Design review of the part shown in the three views and the two pictorial views. Dimensions are in mm from the part's minimum x, y and z. A direction names the side the tool comes from. Round coordinates to 2 decimals unless told otherwise and drop trailing zeros. Loops run counter-clockwise (first coordinate to the right, second up) from the corner with the lowest first, then second, coordinate; pieces in that order, holes last.
1. Consider section A-A on y = 40.85. State the section outline as (x, z) points (3 decimals), then the cut area to 3 significant figures.
2. Consider section D-D on y = 24. State the section outline as (x, z) points, then the cut area to 3 significant figures.
3. Consider section C-C on z = 14.25. State the section outline as (x, y) points.
4. To check wall thickness, follow line 1 along Z through (x, y) = (1.85, 40.85) (3 decimals); line 2 along Z through (x, y) = (109, 2.5); line 3 along Y through (x, z) = (45, 3). State the ranges of each line that lie inside material, in increasing order.
5. Consider section B-B on x = 124. State the section outline as (y, z) points, then the cut area to 3 significant figures.
6. Clearance check with flat-ended pins moving along their axes: pin 1 Ø5 at (y, z) = (12.5, 17) entering from +X; pin 2 Ø4 at (x, y) = (152.5, 8) entering from +Z; pin 3 Ø3 at (x, z) = (37.5, 20.5) entering from +Y. State where each tip first meets the part, or that it passes through.
7. Tool access review of the marked faces 1 and 2: name each direction out of +Z, -Z, +X, -X, +Y, -Y from which nothing blocks a thin tool from reaching the whole face with its end or side.
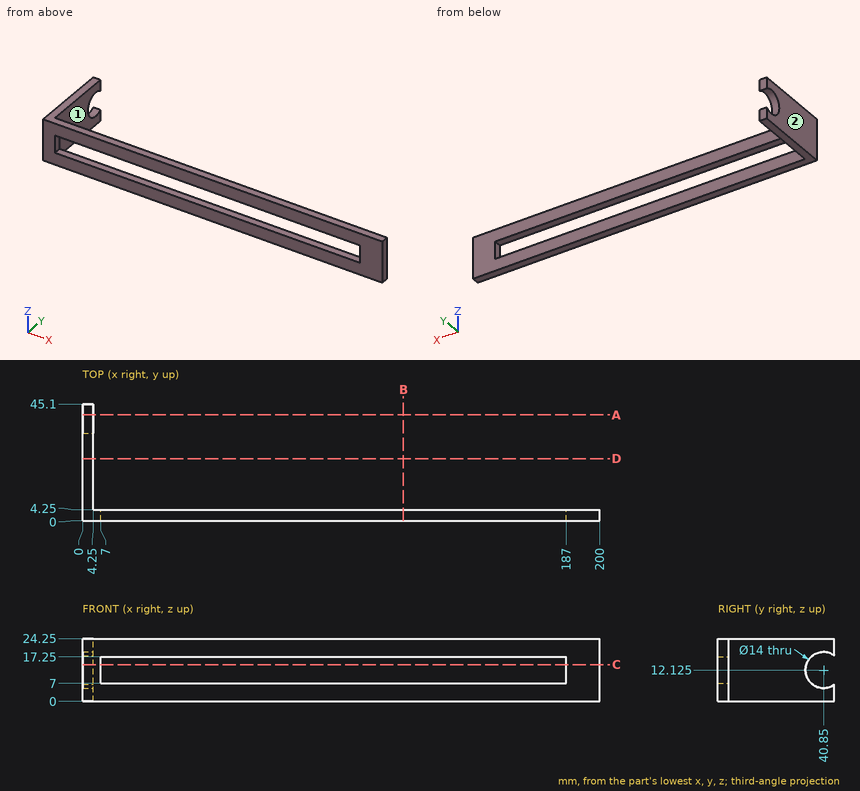
Resolved:
1. outline: (0, 0) - (4.25, 0) - (4.25, 5.125) - (0, 5.125) - close; (0, 19.125) - (4.25, 19.125) - (4.25, 24.25) - (0, 24.25) - close
1. area: 43.6 mm2
2. outline: (0, 0) - (4.25, 0) - (4.25, 24.25) - (0, 24.25) - close
2. area: 103 mm2
3. outline: (0, 0) - (7, 0) - (7, 4.25) - (4.25, 4.25) - (4.25, 34.18) - (0, 34.18) - close; (187, 0) - (200, 0) - (200, 4.25) - (187, 4.25) - close
4. line 1: z = 0 to 5.125, 19.125 to 24.25
4. line 2: z = 0 to 7, 17.25 to 24.25
4. line 3: y = 0 to 4.25
5. outline: (0, 0) - (4.25, 0) - (4.25, 7) - (0, 7) - close; (0, 17.25) - (4.25, 17.25) - (4.25, 24.25) - (0, 24.25) - close
5. area: 59.5 mm2
6. pin 1: stops at x = 4.25
6. pin 2: passes through
6. pin 3: stops at y = 4.25
7. face 1: +Z, -Z, +X, +Y
7. face 2: +Z, -Z, -X, +Y, -Y
